Verification items for the finished model (mm, model axes). Face numbers are marked on the shaded views. A direction names the side the tool comes from. Round coordinates to 2 decimals unless told otherwise and drop trailing zeros. Write each loop counter-clockwise with the first axis right and the second up, starting at its lowest first coordinate (ties: lowest second). Pieces come first, ordered by that corner, then holes. Notation, with made-up numbers: (74, 76.5) -> (94, 76.5) arc R20 cw to (94, 86.5) -> close; hole circle Ø9 at (-0.75, 82). An arc over 180 degrees is marked (long way). Answer as a JSON object with one key per item and string values. Group by question number.
(1) Sectioned sample at A-A on y = 1.25. Record the cut outline in (x, z), and give its area (3 significant figures).
(2) Set-up check for the marked faces 1 and 2: record each of +Z, -Z, +X, -X, +Y, -Y from which the full face is reachable in a straight line by a thin tool's end or side.
(3) Sectioned sample at B-B on z = 2.75. Record the cut outline in (x, y).
(4) Sectioned sample at C-C on x = 8. Record the cut outline in (y, z).
(5) Scan lines: L1, parallel to Y at x = 7, z = 5.5; L2, parallel to Y at x = -13, z = 3; L3, parallel to X at y = 0, z = 2. Record each from-to range of solid material in increasing order. Write a range as from..to.
(6) Gauge pin test, flat end, axial feed: pin 1 Ø1.5 at (y, z) = (-4, 1) entering from -X. Record the tip position at first contact, or that the pin passes through.
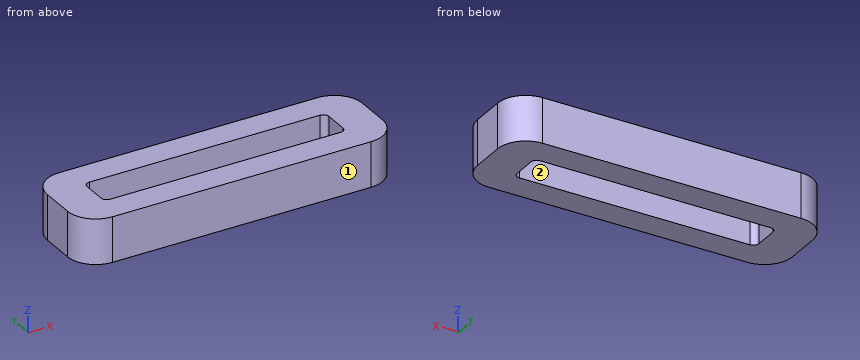
```python
from build123d import *

# Parameters (mm, degrees)
F1_DEPTH = 8


with BuildPart() as f1:
    # F0 (on Top) → F1 (new body)
    with BuildSketch(Plane.XY):
        with BuildLine():
            Line((30.910678, 8.910768), (-15.089322, 8.910768))
            ThreePointArc((-15.089322, 8.910768), (-18.624856, 7.446301), (-20.089322, 3.910768))
            Line((-20.089322, 3.910768), (-20.089322, 0.910768))
            Line((-20.089322, 0.910768), (-20.089322, -2.089232))
            ThreePointArc((-20.089322, -2.089232), (-18.624856, -5.624766), (-15.089322, -7.089232))
            Line((-15.089322, -7.089232), (30.910678, -7.089232))
            ThreePointArc((30.910678, -7.089232), (34.446212, -5.624766), (35.910678, -2.089232))
            Line((35.910678, -2.089232), (35.910678, 0.910768))
            Line((35.910678, 0.910768), (35.910678, 3.910768))
            ThreePointArc((35.910678, 3.910768), (34.446212, 7.446301), (30.910678, 8.910768))
        make_face()
        with BuildLine():
            Line((-13.589322, -1.189232), (-13.589322, 0.910768))
            Line((-13.589322, 0.910768), (-13.589322, 3.010768))
            ThreePointArc((-13.589322, 3.010768), (-13.296429, 3.717874), (-12.589322, 4.010768))
            Line((-12.589322, 4.010768), (28.410678, 4.010768))
            ThreePointArc((28.410678, 4.010768), (29.117785, 3.717874), (29.410678, 3.010768))
            Line((29.410678, 3.010768), (29.410678, 0.910768))
            Line((29.410678, 0.910768), (29.410678, -1.189232))
            ThreePointArc((29.410678, -1.189232), (29.117785, -1.896339), (28.410678, -2.189232))
            Line((28.410678, -2.189232), (-12.589322, -2.189232))
            ThreePointArc((-12.589322, -2.189232), (-13.296429, -1.896339), (-13.589322, -1.189232))
        make_face(mode=Mode.SUBTRACT)
    extrude(amount=F1_DEPTH)


solid = f1.part
```
Computed values:
{
 "1": {"outline": "(-20.09, 0) -> (-13.59, 0) -> (-13.59, 8) -> (-20.09, 8) -> close; (29.41, 0) -> (35.91, 0) -> (35.91, 8) -> (29.41, 8) -> close", "area": "104 mm2"},
 "2": {"face 1": "+Z, -Z, +X, -X, -Y", "face 2": "+Z, -Z"},
 "3": {"outline": "(-20.09, -2.09) arc R5 ccw to (-15.09, -7.09) -> (30.91, -7.09) arc R5 ccw to (35.91, -2.09) -> (35.91, 3.91) arc R5 ccw to (30.91, 8.91) -> (-15.09, 8.91) arc R5 ccw to (-20.09, 3.91) -> close; hole (-13.59, -1.19) arc R1 ccw to (-12.59, -2.19) -> (28.41, -2.19) arc R1 ccw to (29.41, -1.19) -> (29.41, 3.01) arc R1 ccw to (28.41, 4.01) -> (-12.59, 4.01) arc R1 ccw to (-13.59, 3.01) -> close"},
 "4": {"outline": "(-7.09, 0) -> (-2.19, 0) -> (-2.19, 8) -> (-7.09, 8) -> close; (4.01, 0) -> (8.91, 0) -> (8.91, 8) -> (4.01, 8) -> close"},
 "5": {"L1": "-7.09..-2.19, 4.01..8.91", "L2": "-7.09..-2.1, 3.92..8.91", "L3": "-20.09..-13.59, 29.41..35.91"},
 "6": {"pin 1": "x = -19.95"}
}
